```python
from build123d import *
from OCP.BRepFilletAPI import BRepFilletAPI_MakeChamfer

# Parameters (mm, degrees)
EXTRUDE_1_DEPTH = 10
FILLET_1_R      = 0.5
CHAMFER_1_SIZE  = 1
CHAMFER_1_SIZE2 = 0.707106781


with BuildPart() as part:
    # 草图2 → 凸台-拉伸1 (new body)
    with BuildSketch(Plane.XY):
        Polygon((0, 0), (0, 6), (5, 1), (10, 6), (10, 0), align=None)
    extrude(amount=EXTRUDE_1_DEPTH)

    # 圆角1
    fillet_1_edges = [part.edges().sort_by_distance(p)[0] for p in [
        (5, 1, 5),
    ]]
    fillet(fillet_1_edges, radius=FILLET_1_R)

    # 倒角1: one chamfer whose edges measure the first distance from different faces: ONE call of the kernel's chamfer builder (chamfer() names one face for all edges)
    chamfer_1_edges_1 = [part.edges().sort_by_distance(p)[0] for p in [
        (0, 6, 5),
    ]]
    chamfer_1_side_1 = [part.faces().sort_by_distance(p)[0] for p in [
        (2.323223305, 3.676776695, 5),
    ]]
    chamfer_1_edges_2 = [part.edges().sort_by_distance(p)[0] for p in [
        (10, 6, 5),
    ]]
    chamfer_1_side_2 = [part.faces().sort_by_distance(p)[0] for p in [
        (7.676776695, 3.676776695, 5),
    ]]
    chamfer_1 = BRepFilletAPI_MakeChamfer(part.part.solid().wrapped)
    for e in chamfer_1_edges_1:
        chamfer_1.Add(CHAMFER_1_SIZE, CHAMFER_1_SIZE2, e.wrapped, chamfer_1_side_1[0].wrapped)  # the first distance lies on this face
    for e in chamfer_1_edges_2:
        chamfer_1.Add(CHAMFER_1_SIZE, CHAMFER_1_SIZE2, e.wrapped, chamfer_1_side_2[0].wrapped)  # the first distance lies on this face
    add(Compound.cast(chamfer_1.Shape()), mode=Mode.REPLACE)


solid = part.part
```
Check sheet for the modelled part. Datum: model origin and axes. Units: mm. Give positions to 0.01 mm unless a question says otherwise; leave off trailing zeros. Order: outer loops, then holes, each group sorted by start corner. A loop starts at its lowest first (then second) coordinate and runs counter-clockwise, first axis right, second up. Notation, with made-up numbers: (60, -20.5) -> (75, -20.5) arc R26 ccw to (75, -4.5) -> close; hole circle Ø3 at (32, -18.5). An arc over 180 degrees is marked (long way). Use CSV: the item, a comma, the result in double quotes. Start each with the question number.
1) Sectioned sample at A-A, the plane y = 4. Record the boundary of the cut face in (x, z), plus the area to 3 significant figures.
2) Sectioned sample at D-D, the plane x = 4.5. Record the boundary of the cut face in (y, z), plus the area to 3 significant figures.
3) Go/stop test with flat-tipped pins: P1, Ø4, axis at x = 2, z = 1.5, coming from the -Y side; P2, Ø2, axis at x = 5, y = 3.5, coming from the -Z side. Record where each tip stops, or that it passes through.
4) Mould release check, pull along X, two halves, no side actions. Record for faces 1 (the face through (5, 0, 5)), 2 (the face through (0, 3, 5)), 3 (the face through (7, 3, 5)), 4 (the face through (3, 3, 5)): released by +X, released by -X, zero draft, split by the parting line, or undercut.
5) Sectioned sample at B-B, the plane z = 3.5. Record the boundary of the cut face in (x, y).
6) Material ranges on line 1 (X direction, y = 3.05, z = 2.5); line 2 (X direction, y = 3.95, z = 4.5); line 3 (Y direction, x = 5, z = 8), recorded low to high. Write a range as from..to.
7) Sectioned sample at C-C, the plane y = 2.2. Record the boundary of the cut face in (x, z).
Recorded:
1,outline,"(0, 0) -> (2, 0) -> (2, 10) -> (0, 10) -> close; (8, 0) -> (10, 0) -> (10, 10) -> (8, 10) -> close"
1,area,"40.0 mm2"
2,outline,"(0, 0) -> (1.5, 0) -> (1.5, 10) -> (0, 10) -> close"
2,area,"15.0 mm2"
3,P1,"y = 0"
3,P2,"through"
4,face 1,"zero draft"
4,face 2,"released by -X"
4,face 3,"undercut"
4,face 4,"undercut"
5,outline,"(0, 0) -> (10, 0) -> (10, 5.29) -> (9.29, 5.29) -> (5.35, 1.35) arc R0.5 cw to (4.65, 1.35) -> (0.71, 5.29) -> (0, 5.29) -> close"
6,line 1,"0..2.95, 7.05..10"
6,line 2,"0..2.05, 7.95..10"
6,line 3,"0..1.21"
7,outline,"(0, 0) -> (3.8, 0) -> (3.8, 10) -> (0, 10) -> close; (6.2, 0) -> (10, 0) -> (10, 10) -> (6.2, 10) -> close"
